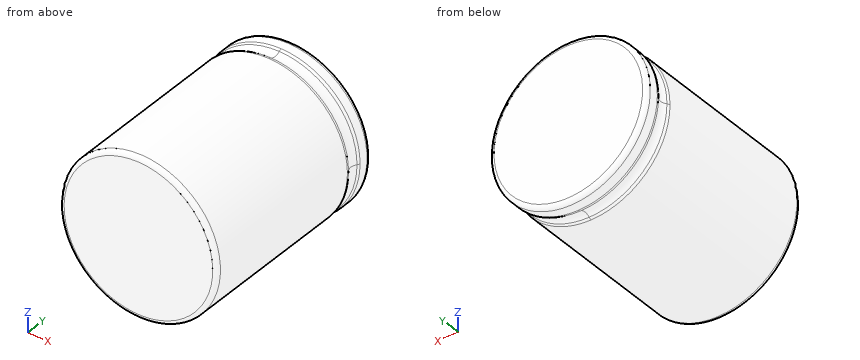
```python
from build123d import *

# Parameters (mm, degrees)
ESBO_O1_R                = 17.85
RESSALTO_EXTRUS_O1_DEPTH = 46
FILETE1_R                = 1
FILETE2_R                = 1


with BuildPart() as part:
    # Esboço1 → Ressalto-extrusão1 (new body)
    with BuildSketch(Plane(origin=(0, 0, 0), x_dir=(1, 0, 0), z_dir=(0, 1, 0))):
        with Locations(Location((0, 0, 0), (0, 0, 270))):
            Circle(ESBO_O1_R)
    extrude(amount=RESSALTO_EXTRUS_O1_DEPTH)

    # Varredura de corte1: sweep along a curve in space
    with BuildLine() as varredura_de_corte1_path:
        ThreePointArc((0, 46, 17.85), (12.621856044, 46, 12.621856044), (17.85, 46, 0))
        ThreePointArc((17.85, 46, 0), (12.621856044, 46, -12.621856044), (0, 46, -17.85))
        ThreePointArc((0, 46, -17.85), (-12.621856044, 46, -12.621856044), (-17.85, 46, 0))
        ThreePointArc((-17.85, 46, 0), (-12.621856044, 46, 12.621856044), (0, 46, 17.85))
    # Esboço2 → Varredura de corte1 (sweep, cut)
    with BuildSketch(Plane.XY):
        with BuildLine():
            Line((17.85, 42.5), (17.85, 39.5))
            ThreePointArc((17.85, 39.5), (17.172875656, 41), (17.85, 42.5))
        make_face()
    sweep(path=varredura_de_corte1_path.line, mode=Mode.SUBTRACT)

    # Filete1
    filete1_edges = [part.edges().sort_by_distance(p)[0] for p in [
        (0, 0, -17.85),
        (0, 46, -17.85),
    ]]
    fillet(filete1_edges, radius=FILETE1_R)

    # Filete2
    filete2_edges = [part.edges().sort_by_distance(p)[0] for p in [
        (12.621856044, 39.5, -12.621856044),
        (12.621856044, 42.5, -12.621856044),
    ]]
    fillet(filete2_edges, radius=FILETE2_R)


solid = part.part
```
Build history of the part. All positions in model axes, mm. Give positions to 0.01 mm unless a question says otherwise; leave off trailing zeros. Loops run counter-clockwise (first coordinate to the right, second up) from the corner with the lowest first, then second, coordinate; pieces in that order, holes last. Notation, with made-up numbers: (83.5, 36.5) - (91.5, 36.5) arc R22 cw to (91.5, 64.5) - close; hole circle Ø6 at (-7.5, -12). An arc over 180 degrees is marked (long way). Use a Markdown table: item, result.
(1) Drop flat-ended pins along their axis: pin 1 Ø4 at (y, z) = (8, 11.5) entering from -X; pin 2 Ø5 at (x, z) = (13, 3.5) entering from -Y; pin 3 Ø10 at (x, y) = (-6.5, 32.5) entering from +Z; pin 4 Ø8 at (y, z) = (29, 11.5) entering from -X. Give the stop position or say it passes through.
Taken from the geometry:
| item | result |
|---|---|
| pin 1 | x = -15.11 |
| pin 2 | y = 0 |
| pin 3 | z = 17.79 |
| pin 4 | x = -16.2 |
(2) Band-saw the part on A-A (y = 27). Give the cut face in (x, z).
Taken from the geometry:
| item | result |
|---|---|
| outline | circle Ø35.7 at (0, 0) |
(3) Wall check: line 1 along Z through (x, y) = (0.5, 3); line 2 along X through (y, z) = (22, 6.5); line 3 along X through (y, z) = (22, -1). Give the ranges that are in metal, low to high.
Taken from the geometry:
| item | result |
|---|---|
| line 1 | -17.84 to 17.84 |
| line 2 | -16.62 to 16.62 |
| line 3 | -17.82 to 17.82 |
